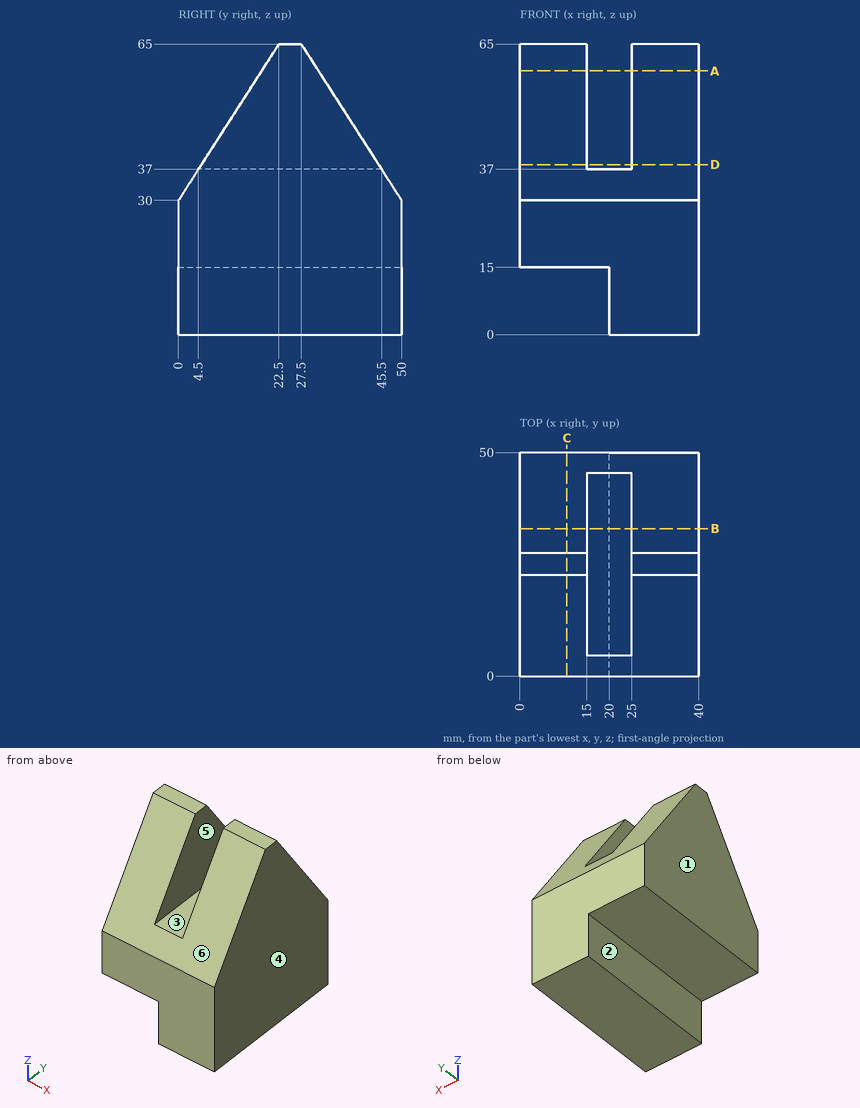
Here's the drawing with two shaded views (mm, measured from the low corner). I have some questions. A direction names the side the tool comes from. Give positions to 0.01 mm unless a question says otherwise; leave off trailing zeros. Loops run counter-clockwise (first coordinate to the right, second up) from the corner with the lowest first, then second, coordinate; pieces in that order, holes last. Notation, with made-up numbers: M 18.5,-18 L 60.5,-18 A29 cw 60.5,3 Z; hole C 12,-7 d8. An arc over 180 degrees is marked long. One line per item, written item: value.
1) Imagine slicing it at B-B on y = 33. Write out the boundary of the cut face in (x, z), and give its area (3 significant figures).
Geometry check:
outline: M 0,15 L 20,15 L 20,0 L 40,0 L 40,56.44 L 25,56.44 L 25,37 L 15,37 L 15,56.44 L 0,56.44 Z
area: 1,760 mm²
2) Imagine slicing it at C-C on x = 10.5. Write out the boundary of the cut face in (y, z).
Geometry check:
outline: M 0,15 L 50,15 L 50,30 L 27.5,65 L 22.5,65 L 0,30 Z
3) Imagine slicing it at A-A on z = 59. Write out the boundary of the cut face in (x, y).
Geometry check:
outline: M 0,18.64 L 15,18.64 L 15,31.36 L 0,31.36 Z; M 25,18.64 L 40,18.64 L 40,31.36 L 25,31.36 Z
4) Please list where these lines run through material, in increasing order: line 1 (X direction, y = 38.5, z = 43); line 2 (X direction, y = 3.5, z = 11); line 3 (Z direction, x = 24.5, y = 37).
Geometry check:
line 1: x = 0 to 15, 25 to 40
line 2: x = 20 to 40
line 3: z = 0 to 37
5) I'm going to push flat-ended pins straight in: pin 1 (12 mm diameter, centred on y = 33, z = 4.5, fed in from -X); pin 2 (1.5 mm diameter, centred on x = 5, y = 16.5, fed in from -Z); pin 3 (5 mm diameter, centred on x = 26.5, z = 36, fed in from -Y). Where does each tip first touch, or does it pass through?
Geometry check:
pin 1: stops at x = 20
pin 2: stops at z = 15
pin 3: stops at y = 2.25
6) Imagine slicing it at D-D on z = 38. Write out the boundary of the cut face in (x, y), and give its area (3 significant figures).
Geometry check:
outline: M 0,5.14 L 15,5.14 L 15,44.86 L 0,44.86 Z; M 25,5.14 L 40,5.14 L 40,44.86 L 25,44.86 Z
area: 1,190 mm²
7) On a 3-axis mill with a long thin cutter (end or side, diameter ignored), from which of +Z, -Z, +X, -X, +Y, -Y can I reach the whole of each face in a straight line? I mean the marked faces 1, 2 and 3. Say none if no direction works.
Geometry check:
face 1: +Z, -Z, -X, +Y, -Y
face 2: -Z, -X, +Y, -Y
face 3: +Z, +Y, -Y
8) Thinking about a two-plate mould opening in X: for the marked faces 4, 5 and 6, which applies, +X half, -X half, draft (parallel to the pull), parting line (faces both ways), or undercut?
Geometry check:
face 4: +X half
face 5: undercut
face 6: draft
